Geometry check sheet. Reference: drawing and pictorial views, mm from the part's lowest x, y, z. A direction names the side the tool comes from. Round coordinates to 2 decimals unless told otherwise and drop trailing zeros. Write each loop counter-clockwise with the first axis right and the second up, starting at its lowest first coordinate (ties: lowest second). Pieces come first, ordered by that corner, then holes. Notation, with made-up numbers: (79, 38.25) -> (92, 38.25) arc R21 cw to (92, 47.25) -> close; hole circle Ø1 at (-30.5, 39.5). An arc over 180 degrees is marked (long way). Write item = value, one per line.
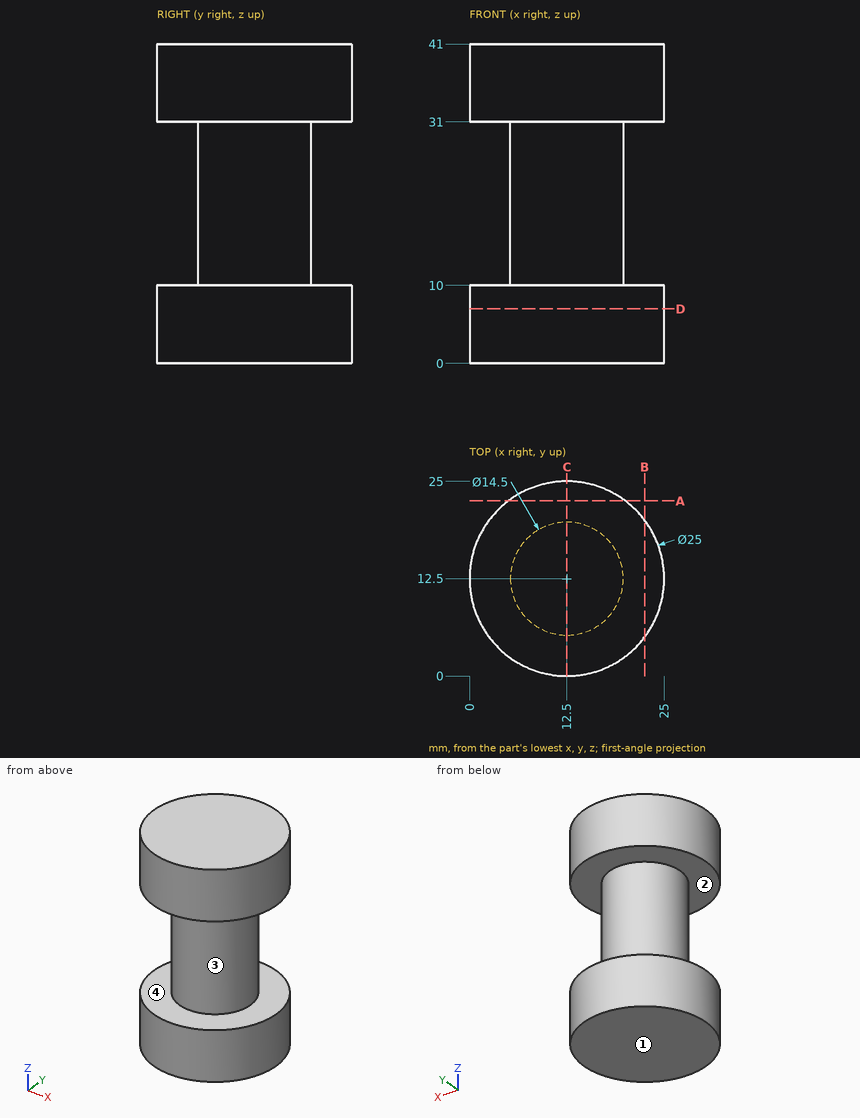
(1) Sectioned sample at C-C on x = 12.5. Enter the section's corners in (y, z), then the cut area to 4 significant figures.
Worked answers:
outline = (0, 0) -> (25, 0) -> (25, 10) -> (19.75, 10) -> (19.75, 31) -> (25, 31) -> (25, 41) -> (0, 41) -> (0, 31) -> (5.25, 31) -> (5.25, 10) -> (0, 10) -> close
area = 804.5 mm²
(2) Material ranges on L1, parallel to Z at x = 19.25, y = 20.5; L2, parallel to X at y = 16, z = 11.5; L3, parallel to X at y = 6.25, z = 12, recorded low to high. Write a range as [from, to].
Worked answers:
L1 = [0, 10], [31, 41]
L2 = [6.15, 18.85]
L3 = [8.83, 16.17]
(3) Release check for a two-part mould opening along X. For the marked faces 3 and 4 record: pulls with the +X half, pulls with the -X half, needs draft (parallel to the pull), parting line crosses it, or undercut.
Worked answers:
face_3 = parting line crosses it
face_4 = needs draft
(4) Access from +Z, -Z, +X, -X, +Y, -Y to the whole of each face (thin tool, end or side, straight path). Record for the marked faces 1 and 2.
Worked answers:
face_1 = -Z, +X, -X, +Y, -Y
face_2 = none
(5) Sectioned sample at D-D on z = 7. Enter the section's corners in (x, y).
Worked answers:
outline = circle Ø25 at (12.5, 12.5)
(6) Go/stop test with flat-tipped pins: P1, Ø5, axis at y = 18, z = 7.5, coming from the -X side; P2, Ø10, axis at x = 7.5, z = 19, coming from the +Y side; P3, Ø1, axis at y = 13, z = 30, coming from the -X side. Record where each tip stops, or that it passes through.
Worked answers:
P1 = 0.37
P2 = 19.75
P3 = 5.25
(7) Sectioned sample at A-A on y = 22.5. Enter the section's corners in (x, z), then the cut area to 3 significant figures.
Worked answers:
outline = (5, 0) -> (20, 0) -> (20, 10) -> (5, 10) -> close; (5, 31) -> (20, 31) -> (20, 41) -> (5, 41) -> close
area = 300 mm²
